from build123d import *

# Parameters (mm, degrees)
SKETCH1_W               = 141.842971217
SKETCH1_H               = 108.306454767
BOSS_EXTRUDE1_DEPTH     = 5
BOSS_EXTRUDE2_DEPTH     = 95
SKETCH3_W               = 111.927402264
SKETCH3_H               = 61.729715964
CUT_EXTRUDE1_DEPTH      = 95
SKETCH4_W               = 61.729715964
SKETCH4_H               = 100
CUT_EXTRUDE2_DEPTH      = 95
SKETCH5_W               = 141.842971217
SKETCH5_H               = 26.901252983
CUT_EXTRUDE3_DEPTH      = 135
BOSS_EXTRUDE3_DEPTH     = 5
CUT_EXTRUDE4_DEPTH      = 65
CUT_EXTRUDE4_DEPTH_BACK = 15


with BuildPart() as part:
    # Sketch1 → Boss-Extrude1 (new body)
    with BuildSketch(Plane(origin=(0, 0, 22.06567104), x_dir=(1, 0, 0), z_dir=(0, 1, 0))):
        with Locations((16.768258226, -27.626392649)):
            Rectangle(SKETCH1_W, SKETCH1_H)
    extrude(amount=BOSS_EXTRUDE1_DEPTH)

    # Sketch2 → Boss-Extrude2 (add)
    with BuildSketch(Plane(origin=(0, 5, 22.06567104), x_dir=(1, 0, 0), z_dir=(0, 1, 0))):
        Polygon((-54.153227383, -81.779620033), (87.689743834, -81.779620033), (87.689743834, -44.802673151), (87.689743834, 26.526834734), (57.774174881, 26.526834734), (-54.153227383, 26.526834734), (-54.153227383, 16.927042813), (57.774174881, 16.927042813), (57.774174881, -44.802673151), (-54.153227383, -44.802673151), align=None)
    extrude(amount=BOSS_EXTRUDE2_DEPTH)

    # Sketch3 → Cut-Extrude1 (cut)
    with BuildSketch(Plane(origin=(0, 5, 22.06567104), x_dir=(1, 0, 0), z_dir=(0, 1, 0))):
        with Locations((1.810473749, -13.937815169)):
            Rectangle(SKETCH3_W, SKETCH3_H)
    extrude(amount=-CUT_EXTRUDE1_DEPTH, mode=Mode.SUBTRACT)

    # Sketch4 → Cut-Extrude2 (cut)
    with BuildSketch(Plane(origin=(57.774174881, 0, 22.06567104), x_dir=(0, 0, 1), z_dir=(-1, 0, 0))):
        with Locations((13.937815169, 50)):
            Rectangle(SKETCH4_W, SKETCH4_H)
    extrude(amount=-CUT_EXTRUDE2_DEPTH, mode=Mode.SUBTRACT)


with BuildPart() as cut_extrude2_piece_1:
    # of the separate pieces the step leaves, piece 1, a body of its own (cut_extrude2_pieces)
    add(part.part.solids().sort_by_distance((-54.153227383, 100, 66.868344191))[0])

    # Sketch5 → Cut-Extrude3 (cut)
    with BuildSketch(Plane(origin=(0, 100, 0), x_dir=(1, 0, 0), z_dir=(0, 1, 0))):
        with Locations((16.768258226, -80.318970683)):
            Rectangle(SKETCH5_W, SKETCH5_H)
    extrude(amount=-CUT_EXTRUDE3_DEPTH, mode=Mode.SUBTRACT)



with BuildPart() as cut_extrude2_piece_2:
    # of the separate pieces the step leaves, piece 2, a body of its own (cut_extrude2_pieces)
    add(part.part.solids().sort_by_distance((-54.153227383, 0, -4.461163693))[0])


with BuildPart() as cut_extrude2_piece_1_1:
    add(cut_extrude2_piece_1.part)

    add(cut_extrude2_piece_2.part)  # Boss-Extrude3 merges Cut-Extrude2 piece 2
    # Sketch6 → Boss-Extrude3 (add)
    with BuildSketch(Plane(origin=(0, 100, 0), x_dir=(1, 0, 0), z_dir=(0, 1, 0))):
        Polygon((87.689743834, -103.845291074), (87.689743834, 4.461163693), (75.84574379, 4.461163693), (75.84574379, -13.640842184), (-46.610502058, -13.640842184), (-51.612768373, -17.284729089), (-46.610502058, -20.928615994), (75.84574379, -20.928615994), (75.84574379, -37.985107889), (-46.610502058, -37.985107889), (-51.612768373, -41.008758725), (-46.610502058, -44.032409561), (75.84574379, -44.032409561), (75.84574379, -51.94041944), (-46.610502058, -51.94041944), (-51.612768373, -55.584306345), (-47.3197879, -59.22819325), (75.84574379, -59.22819325), (75.84574379, -70.082324456), (-46.610502058, -70.082324456), (-51.612768373, -73.416093326), (-47.3197879, -76.749862197), (75.84574379, -76.749862197), (75.84574379, -103.845291074), align=None)
    extrude(amount=-BOSS_EXTRUDE3_DEPTH)

    # Sketch7 → Cut-Extrude4 (cut, two sides: drawn at the far end of the back side and taken through both)
    with BuildSketch(Plane.XY.offset(20.928615994).offset(-CUT_EXTRUDE4_DEPTH_BACK)):
        Polygon((-51.612768373, 100), (-26.03457971, 95), (-51.612768373, 95), align=None)
    extrude(amount=CUT_EXTRUDE4_DEPTH + CUT_EXTRUDE4_DEPTH_BACK, mode=Mode.SUBTRACT)


solid = cut_extrude2_piece_1_1.part
Part model, mm, in its own coordinate system. A direction names the side the tool comes from. Coordinates: 2 decimals unless noted, no trailing zeros. Write each loop counter-clockwise with the first axis right and the second up, starting at its lowest first coordinate (ties: lowest second). Pieces come first, ordered by that corner, then holes. Notation, with made-up numbers: M 88,-36 L 134,-36 A35 cw 134,-3 Z; hole C -37,55.25 d2. An arc over 180 degrees is marked long. Return JSON: item names as keys, results as strings.
1. Flat gauge pin, fed straight in: pin 1 Ø4 at (y, z) = (98.5, 33.5) entering from -X. Where does the tip first touch, or does it go through?
Determined:
{"pin 1": "x = 75.85"}
2. Saw through at D-D, the plane z = 85. Write the cut outline in (x, y).
Determined:
{"outline": "M 75.85,95 L 87.69,95 L 87.69,100 L 75.85,100 Z"}
3. 3-axis set-ups, long thin cutter, end or side, ignore diameter. For faces 4 (the face through (-39.003, 97.535, 73.369)), 5 (the face through (75.846, 98, 29)), 6 (the face through (87.69, 53, 94)): which of +Z, -Z, +X, -X, +Y, -Y reach the whole face in a straight line?
Determined:
{"face 4": "-X, -Y", "face 5": "-X, +Y, -Y", "face 6": "+Z, -Z, +X, +Y, -Y"}
4. Probe L1, parallel to Z at x = 27.5, y = 85.5; L2, parallel to Y at x = 58.5, z = 40; L3, parallel to Y at x = -32, z = 19. List the from-to ranges inside material, lowest first.
Determined:
{"L1": "-4.46 to 5.14, 93.77 to 103.85", "L2": "95 to 100", "L3": "96.17 to 100"}
5. Pull direction Z, two halves, no side cores. Call faces 1 (the face through (13, 98, 59.228)), 2 (the face through (18, 49, -4.461)), 3 (the face through (-54.153, 49, 0)): pulls with the +Z half, pulls with the -Z half, needs draft (parallel to the pull), parting line crosses it, or undercut.
Determined:
{"face 1": "undercut", "face 2": "pulls with the -Z half", "face 3": "needs draft"}
6. Saw through at C-C, the plane x = -33. Write the cut outline in (y, z).
Determined:
{"outline": "M 0,-4.46 L 100,-4.46 L 100,5.14 L 0,5.14 Z; M 0,93.77 L 100,93.77 L 100,103.85 L 0,103.85 Z; M 96.36,13.64 L 100,13.64 L 100,20.93 L 96.36,20.93 Z; M 96.36,37.99 L 100,37.99 L 100,44.03 L 96.36,44.03 Z; M 96.36,51.94 L 100,51.94 L 100,59.23 L 96.36,59.23 Z; M 96.36,70.08 L 100,70.08 L 100,76.75 L 96.36,76.75 Z"}
7. Saw through at B-B, the plane y = 34.5. Write the cut outline in (x, z).
Determined:
{"outline": "M -54.15,-4.46 L 87.69,-4.46 L 87.69,5.14 L -54.15,5.14 Z; M -54.15,93.77 L 87.69,93.77 L 87.69,103.85 L -54.15,103.85 Z"}
8. Saw through at A-A, the plane x = 27. Write the cut outline in (y, z).
Determined:
{"outline": "M 0,-4.46 L 100,-4.46 L 100,5.14 L 0,5.14 Z; M 0,93.77 L 100,93.77 L 100,103.85 L 0,103.85 Z; M 95,13.64 L 100,13.64 L 100,20.93 L 95,20.93 Z; M 95,37.99 L 100,37.99 L 100,44.03 L 95,44.03 Z; M 95,51.94 L 100,51.94 L 100,59.23 L 95,59.23 Z; M 95,70.08 L 100,70.08 L 100,76.75 L 95,76.75 Z"}
